Check sheet for the modelled part. Datum: model origin and axes. Units: mm. A direction names the side the tool comes from. Give positions to 0.01 mm unless a question says otherwise; leave off trailing zeros. Order: outer loops, then holes, each group sorted by start corner. A loop starts at its lowest first (then second) coordinate and runs counter-clockwise, first axis right, second up.
Autodesk Inventor part; units mm, degrees
ref_plane "YZ Plane" through (0, 0, 0) normal (1, 0, 0) x (0, 1, 0)
ref_plane "XZ Plane" through (0, 0, 0) normal (0, 1, 0) x (-1, 0, 0)
ref_plane "XY Plane" through (0, 0, 0) normal (0, 0, 1) x (1, 0, 0)
sketch "Sketch1" plane through (0, 0, 0) normal (0, 1, 0) x (-1, 0, 0)
  line L0 (-15.5, 17.5) -> (15.5, 17.5)
  line L1 (17.5, 15.5) -> (17.5, -15.5)
  line L2 (15.5, -17.5) -> (-15.5, -17.5)
  line L3 (-17.5, -15.5) -> (-17.5, 15.5)
  line L4 (-17.5, 17.5) -> (17.5, -17.5) construction
  line L5 (17.5, 17.5) -> (-17.5, -17.5) construction
  line L6 (-13.9, -15.9) -> (13.9, -15.9)
  line L7 (15.9, -13.9) -> (15.9, 13.9)
  line L8 (13.9, 15.9) -> (-13.9, 15.9)
  line L9 (-15.9, 13.9) -> (-15.9, -13.9)
  arc A0 (17.5, 15.5) -> (15.5, 17.5) centre (15.5, 15.5) ccw
  arc A1 (15.5, -17.5) -> (17.5, -15.5) centre (15.5, -15.5) ccw
  arc A2 (-17.5, -15.5) -> (-15.5, -17.5) centre (-15.5, -15.5) ccw
  arc A3 (-15.5, 17.5) -> (-17.5, 15.5) centre (-15.5, 15.5) ccw
  arc A4 (15.9, 13.9) -> (13.9, 15.9) centre (13.9, 13.9) ccw
  arc A5 (13.9, -15.9) -> (15.9, -13.9) centre (13.9, -13.9) ccw
  arc A6 (-15.9, -13.9) -> (-13.9, -15.9) centre (-13.9, -13.9) ccw
  arc A7 (-13.9, 15.9) -> (-15.9, 13.9) centre (-13.9, 13.9) ccw
  point P0 (0, 0)
  dimension "d0" = 35
  dimension "d1" = 35
  dimension "d2" = 1.6
  dimension "d3" = 2
extrude "Extrusion1" add sketch "Sketch1" along normal blind 100
properties part number "AlignmentTube" material "Steel, Mild"
(1) Sectioned sample at A-A (x = 7). Enter the section's corners in (y, z), plus the area to 3 significant figures.
(2) Go/stop test with a flat-tipped pin: P1, Ø12, axis at x = 10.5, z = 10.5, coming from the +Y side. Record where the tip stops, or that it passes through.
(3) Sectioned sample at C-C (y = 59). Enter the section's corners in (x, z), plus the area to 3 significant figures.
(4) Sectioned sample at B-B (z = -3). Enter the section's corners in (x, y).
(5) Thickness scan on L1, parallel to Z at x = 3, y = 18; L2, parallel to Z at x = 15.5, y = 25. Record the ranges inside material, lowest first.
(6) Release check for a two-part mould opening along X. For faces 1 (the face through (0, 100, -17)), 2 (the face through (16.9, 49.3, -16.93)), 3 (the face through (15.9, 49, 0)) record: released by +X, released by -X, zero draft, split by the parting line, or undercut.
(7) Tool access check on faces 4 (the face through (0, 49, -15.9)), 5 (the face through (0, 49, 17.5)). Record the directions out of +Z, -Z, +X, -X, +Y, -Y that give a thin tool (end or side, any length) a straight path to the whole face; none if there is none.
Values follow:
1. outline: (0, -17.5) - (100, -17.5) - (100, -15.9) - (0, -15.9) - close; (0, 15.9) - (100, 15.9) - (100, 17.5) - (0, 17.5) - close
1. area: 320 mm2
2. P1: stops at y = 100
3. outline: (-17.5, -15.5) arc R2 ccw to (-15.5, -17.5) - (15.5, -17.5) arc R2 ccw to (17.5, -15.5) - (17.5, 15.5) arc R2 ccw to (15.5, 17.5) - (-15.5, 17.5) arc R2 ccw to (-17.5, 15.5) - close; hole (-15.9, -13.9) arc R2 ccw to (-13.9, -15.9) - (13.9, -15.9) arc R2 ccw to (15.9, -13.9) - (15.9, 13.9) arc R2 ccw to (13.9, 15.9) - (-13.9, 15.9) arc R2 ccw to (-15.9, 13.9) - close
3. area: 214 mm2
4. outline: (-17.5, 0) - (-15.9, 0) - (-15.9, 100) - (-17.5, 100) - close; (15.9, 0) - (17.5, 0) - (17.5, 100) - (15.9, 100) - close
5. L1: z = -17.5 to -15.9, 15.9 to 17.5
5. L2: z = -17.5 to -15.1, 15.1 to 17.5
6. face 1: zero draft
6. face 2: released by +X
6. face 3: undercut
7. face 4: +Y, -Y
7. face 5: +Z, +X, -X, +Y, -Y
